For this review, take the finished solid that the model builds, in its own axes (mm). Face numbers are marked on the shaded views. A direction names the side the tool comes from. Give positions to 0.01 mm unless a question says otherwise; leave off trailing zeros. Order: outer loops, then holes, each group sorted by start corner. A loop starts at its lowest first (then second) coordinate and runs counter-clockwise, first axis right, second up.
Item 1: Consider section D-D (z = 6.5). Give the boundary of the cut face in (x, y).
Item 2: Consider section B-B (z = 1). Give the boundary of the cut face in (x, y), plus the area to 3 significant figures.
Item 3: Machinability: for the marked faces 1, 2, 3 and 4, which of the approach directions +Z, -Z, +X, -X, +Y, -Y give a long, thin tool a straight path to every point of the face, cutting with its end or side? Answer none if there is none.
Item 4: For P1, Ø2, axis at x = 29, z = 2, coming from the -Y side; P2, Ø1.5, axis at y = -4, z = 5.5, coming from the -X side; P3, Ø3, axis at x = 29.5, z = 5, coming from the +Y side; P4, Ø2, axis at x = -3, y = -3.72, coming from the -Z side, all flat-tipped, find the tip position at first contact; note any pin that passes through.
Item 5: Consider section A-A (x = -3). Give the boundary of the cut face in (y, z), plus the area to 3 significant figures.
Item 6: For probe 1 along Y at (x, z) = (-3, 2.85); probe 2 along X at (y, z) = (-4.75, 2.25); probe 3 along Y at (x, z) = (-12, 2.25), list the stretches that pass through material, from the lowest coordinate up.
Item 7: Consider section C-C (y = -1). Give the boundary of the cut face in (x, z).
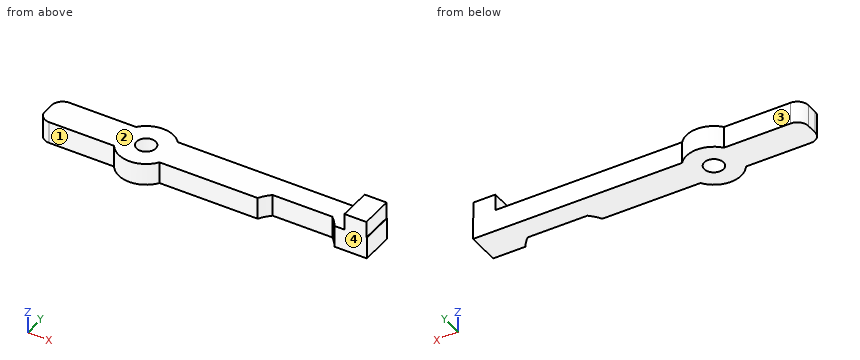
Autodesk Inventor part; units mm, degrees
ref_plane "YZ Plane" through (0, 0, 0) normal (1, 0, 0) x (0, 1, 0)
ref_plane "XZ Plane" through (0, 0, 0) normal (0, 1, 0) x (-1, 0, 0)
ref_plane "XY Plane" through (0, 0, 0) normal (0, 0, 1) x (1, 0, 0)
sketch "Skizze1" plane through (0, 0, 0) normal (0, 0, 1) x (1, 0, 0)
  line L0 (2, -8) -> (-6, -8) construction
  line L1 (2, 0) -> (2, -8) construction
  line L2 (0, 0) -> (2, 0) construction
  line L3 (0, 1.7577) -> (0, 0) construction
  line L4 (2, 1.7577) -> (0, 1.7577) construction
  line L5 (2, 1.7577) -> (2, 8.4467) construction
  line L6 (0, 8.4467) -> (2, 8.4467) construction
  line L7 (0, 11) -> (0, 8.4467) construction
  line L8 (-6, 11) -> (0, 11) construction
  line L9 (-6, -8) -> (-6, 11) construction
  circle A0 centre (-3, -3.7188) radius 1.75 construction
  circle A1 centre (-3, -3.7188) radius 1.75
  line L10 (5.65, 17) -> (8.35, 17) construction
  line L11 (11, -0.5) -> (11, 14.5) construction
  line L12 (3, -0.5) -> (11, -0.5) construction
  line L13 (3, -0.5) -> (3, 14.5) construction
  line L14 (7, 17) -> (39, 17) construction
  line L15 (0.8261, -0.5) -> (39, -0.5)
  line L16 (39, -0.5) -> (39, -6.5)
  line L17 (39, -6.5) -> (1.1551, -6.5)
  line L18 (-6.8261, -0.5) -> (-21, -0.5)
  line L19 (-21, -0.5) -> (-21, -6.5)
  line L20 (-21, -6.5) -> (-7.1551, -6.5)
  line L21 (-6, -6.5) -> (-6, -0.5) construction
  arc A2 (0.8261, -0.5) -> (-6.8261, -0.5) centre (-3, -3.7188) ccw
  arc A3 (-7.1551, -6.5) -> (1.1551, -6.5) centre (-3, -3.7188) ccw
  dimension "d0" = 32
  dimension "d1" = 6
  dimension "d2" = 15
extrude "Extrusion1" add sketch "Skizze1" along normal blind 4
sketch "Skizze2" plane through (1.1551, -6.5, 0) normal (0, -1, 0) x (1, 0, 0)
  line L0 (37.7621, 0) -> (33.7621, 0)
  line L1 (33.7621, 0) -> (33.7621, 7)
  line L2 (33.7621, 7) -> (37.7621, 7)
  line L3 (37.7621, 7) -> (37.7621, 0)
  point P0 (-1.1551, 0)
  dimension "d5" = 4
  dimension "d6" = 7
extrude "Extrusion3" add sketch "Skizze2" against normal blind 6
sketch "Skizze3" plane through (0, 0, 4) normal (0, 0, 1) x (1, 0, 0)
  circle A0 centre (-3, -3.7188) radius 1.75 construction
  line L0 (34.9172, -6.5) -> (34.9172, -0.5) construction
  line L1 (34.9172, -0.5) -> (0.8261, -0.5) construction
  arc A1 (0.8261, -0.5) -> (-6.8261, -0.5) centre (-3, -3.7188) ccw construction
  line L2 (-6.8261, -0.5) -> (-21, -0.5) construction
  line L3 (-21, -0.5) -> (-21, -6.5) construction
  line L4 (-21, -6.5) -> (-7.1551, -6.5) construction
  arc A2 (-7.1551, -6.5) -> (1.1551, -6.5) centre (-3, -3.7188) ccw construction
  line L5 (1.1551, -6.5) -> (34.9172, -6.5) construction
  line L6 (34.9172, -4.4009) -> (29.9172, -4.4009) construction
  arc A3 (33.0892, -6.5) -> (19.0718, -6.5) centre (26.0805, -10.6676) ccw
  line L7 (19.0718, -6.5) -> (33.0892, -6.5)
  line L8 (1.1551, -6.5) -> (34.9172, -6.5) construction
  point P0 (0, 0)
  dimension "d11" = 5
extrude "Extrusion4" cut sketch "Skizze3" against normal blind 6
sketch "Skizze4" plane through (0, 0, 4) normal (0, 0, 1) x (1, 0, 0)
  arc A0 (33.0892, -6.5) -> (19.0718, -6.5) centre (26.0805, -10.6676) ccw construction
  line L0 (33.0892, -6.5) -> (34.9172, -6.5) construction
  line L1 (34.9172, -6.5) -> (34.9172, -0.5) construction
  line L2 (34.9172, -0.5) -> (0.8261, -0.5) construction
  arc A1 (0.8261, -0.5) -> (-6.8261, -0.5) centre (-3, -3.7188) ccw construction
  line L3 (-6.8261, -0.5) -> (-21, -0.5) construction
  line L4 (-21, -0.5) -> (-21, -6.5) construction
  line L5 (-21, -6.5) -> (-7.1551, -6.5) construction
  arc A2 (-7.1551, -6.5) -> (1.1551, -6.5) centre (-3, -3.7188) ccw construction
  line L6 (1.1551, -6.5) -> (19.0718, -6.5) construction
  circle A3 centre (-3, -3.7188) radius 1.75 construction
  line L7 (17.8717, -0.5) -> (33.0892, -0.5)
  line L8 (33.0892, -0.5) -> (33.0892, -4.6064)
  line L9 (33.0892, -4.6064) -> (17.8717, -4.6064)
  line L10 (17.8717, -4.6064) -> (17.8717, -0.5)
  point P0 (0, 0)
extrude "Extrusion5" add sketch "Skizze4" against normal blind 4
fillet "Rundung1" radius 2 2 edges at (-21, -0.5, 2) (-21, -6.5, 2)
properties part number "Reset_beam"
Resolved:
1. outline: (34.92, -6.5) - (38.92, -6.5) - (38.92, -0.5) - (34.92, -0.5) - close
2. outline: (-21, -4.5) arc R2 ccw to (-19, -6.5) - (-7.16, -6.5) arc R5 ccw to (1.16, -6.5) - (19.07, -6.5) arc R8.15 cw to (20.63, -4.61) - (31.54, -4.61) arc R8.15 cw to (33.09, -6.5) - (39, -6.5) - (39, -0.5) - (0.83, -0.5) arc R5 ccw to (-6.83, -0.5) - (-19, -0.5) arc R2 ccw to (-21, -2.5) - close; hole circle Ø3.5 at (-3, -3.72)
2. area: 347 mm2
3. face 1: +Z, -Z, -X, -Y
3. face 2: +Z, -X, +Y, -Y
3. face 3: +Z, -Z, -X, +Y
3. face 4: +Z, -Z, +X, -Y
4. P1: stops at y = -4.61
4. P2: stops at x = 34.92
4. P3: stops at y = -0.5
4. P4: passes through
5. outline: (-8.72, 0) - (-5.47, 0) - (-5.47, 4) - (-8.72, 4) - close; (-1.97, 0) - (1.28, 0) - (1.28, 4) - (-1.97, 4) - close
5. area: 26.0 mm2
6. probe 1: y = -8.72 to -5.47, -1.97 to 1.28
6. probe 2: x = -20.98 to -4.41, -1.59 to 20.47, 31.69 to 39
6. probe 3: y = -6.5 to -0.5
7. outline: (-20.32, 0) - (39, 0) - (39, 4) - (38.92, 4) - (38.92, 7) - (34.92, 7) - (34.92, 4) - (-20.32, 4) - close
